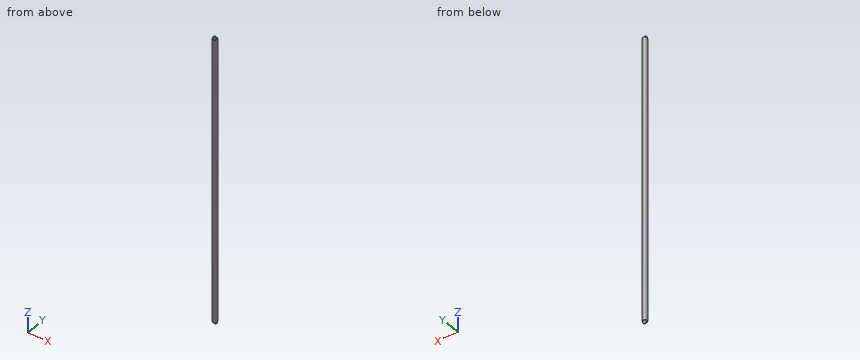
from build123d import *

# Parameters (mm, degrees)
F0_R     = 9.5
F0_R_2   = 7.9
F1_DEPTH = 600
F2_R     = 9.5
F3_DEPTH = 1.6
F4_DEPTH = 1.6


with BuildPart() as f1:
    # F0 (on Top) → F1 (new body)
    with BuildSketch(Plane.XY):
        Circle(F0_R)
        Circle(F0_R_2, mode=Mode.SUBTRACT)
    extrude(amount=F1_DEPTH)

    # F2 (on Front) → F3 (join)
    with BuildSketch(Plane.XZ):
        Circle(F2_R)
    extrude(amount=F3_DEPTH)

    # F3_face (on face) → F4 (join)
    with BuildSketch(Plane(origin=(0, 0, -0.084371), x_dir=(1, 0, 0), z_dir=(0, 1, 0))):
        with BuildLine():
            ThreePointArc((9.5, -0.084371), (0, 9.415629), (-9.5, -0.084371))
            Line((-9.5, -0.084371), (-7.9, -0.084371))
            Line((-7.9, -0.084371), (-7.9, -5.360733))
            ThreePointArc((-7.9, -5.360733), (0, -9.584371), (7.9, -5.360733))
            Line((7.9, -5.360733), (7.9, -0.084371))
            Line((7.9, -0.084371), (9.5, -0.084371))
        make_face()
    extrude(amount=F4_DEPTH)

    # F5: F1 across face


with BuildPart() as f1_1:
    add(f1.part)
    add(f1.part.mirror(Plane.XY.offset(600)))


solid = f1_1.part
CAD build for the part. Positions are in the model's coordinates, mm. Coordinates: 2 decimals unless noted, no trailing zeros. Write each loop counter-clockwise with the first axis right and the second up, starting at its lowest first coordinate (ties: lowest second). Pieces come first, ordered by that corner, then holes. Notation, with made-up numbers: (-23, 54) - (-7, 54) arc R11 ccw to (-7, 66) - close; hole circle Ø7 at (55.25, 84). An arc over 180 degrees is marked (long way). Use a Markdown table: item, result. Add a question column.
Item 1: Drill centre lines: L1, parallel to X at y = 0.5, z = 901; L2, parallel to Y at x = 1.5, z = 674; L3, parallel to Y at x = 2.5, z = 254.5. Where is each one in solid material? Low to high. Write a range as from..to.
Item 2: Flat gauge pins, fed straight in: pin 1 (2.5 mm diameter, centred on x = -3.5, y = -6, fed in from -Z); pin 2 (6 mm diameter, centred on x = 6.5, z = 269.5, fed in from +Y); pin 3 (4 mm diameter, centred on x = -7.5, y = -5.5, fed in from +Z); pin 4 (5.5 mm diameter, centred on x = 1.5, z = -2, fed in from +Y). Where does each tip first touch, or does it go through?
Item 3: Band-saw the part on B-B, the plane z = 899.5. Give the cut face in (x, y), and give its area (3 significant figures).
Item 4: Band-saw the part on A-A, the plane x = 0. Give the cut face in (y, z), and give its area (3 significant figures).
Numbers:
| question | item | result |
|---|---|---|
| 1 | L1 | -9.49..-7.88, 7.88..9.49 |
| 1 | L2 | -9.38..-7.76, 7.76..9.38 |
| 1 | L3 | -9.17..-7.49, 7.49..9.17 |
| 2 | pin 1 | z = 0 |
| 2 | pin 2 | y = 8.83 |
| 2 | pin 3 | z = 1200 |
| 2 | pin 4 | y = 9.5 |
| 3 | outline | circle Ø19 at (0, 0); hole circle Ø15.8 at (0, 0) |
| 3 | area | 87.5 mm2 |
| 4 | outline | (-9.5, 0) - (-7.9, 0) - (-7.9, 1200) - (-9.5, 1200) - close; (-1.6, -9.5) - (1.6, -9.5) - (1.6, 9.5) - (-1.6, 9.5) - close; (-1.6, 1190.5) - (1.6, 1190.5) - (1.6, 1209.5) - (-1.6, 1209.5) - close; (7.9, 0) - (9.5, 0) - (9.5, 1200) - (7.9, 1200) - close |
| 4 | area | 3,960 mm2 |
